Can you work these out from the model? Positions are in its coordinate system, mm. A direction names the side the tool comes from. Give positions to 0.01 mm unless a question says otherwise; leave off trailing zeros. Order: outer loops, then holes, each group sorted by start corner. A loop starts at its lowest first (then second) coordinate and runs counter-clockwise, first axis right, second up. Notation, with made-up numbers: (58.5, 44.25) - (84.5, 44.25) arc R12 ccw to (84.5, 62.25) - close; hole circle Ø4 at (-30, 40.5). An arc over 180 degrees is marked (long way). Answer as a JSON object with one key per item and string values.
```python
from build123d import *

# Parameters (mm, degrees)
SKETCH_1_R      = 45.75
SKETCH_1_R_2    = 1.5
EXTRUDE_1_DEPTH = 4


with BuildPart() as part:
    # 草图1 → 凸台-拉伸1 (new body)
    with BuildSketch(Plane(origin=(0, 0, 0), x_dir=(1, 0, 0), z_dir=(0, 1, 0))):
        with BuildLine():
            Line((-60, -10.5), (-60, 10.5))
            ThreePointArc((-60, 10.5), (-59.560660172, 11.560660172), (-58.5, 12))
            Line((-58.5, 12), (-54.863466897, 12))
            ThreePointArc((-54.863466897, 12), (-53.938159008, 12.31940468), (-53.406914679, 13.14159292))
            ThreePointArc((-53.406914679, 13.14159292), (0, 55), (53.406914679, 13.14159292))
            ThreePointArc((53.406914679, 13.14159292), (53.938159008, 12.31940468), (54.863466897, 12))
            Line((54.863466897, 12), (58.5, 12))
            ThreePointArc((58.5, 12), (59.560660172, 11.560660172), (60, 10.5))
            Line((60, 10.5), (60, -10.5))
            ThreePointArc((60, -10.5), (59.560660172, -11.560660172), (58.5, -12))
            Line((58.5, -12), (54.863466897, -12))
            ThreePointArc((54.863466897, -12), (53.938159008, -12.31940468), (53.406914679, -13.14159292))
            ThreePointArc((53.406914679, -13.14159292), (0, -55), (-53.406914679, -13.14159292))
            ThreePointArc((-53.406914679, -13.14159292), (-53.938159008, -12.31940468), (-54.863466897, -12))
            Line((-54.863466897, -12), (-58.5, -12))
            ThreePointArc((-58.5, -12), (-59.560660172, -11.560660172), (-60, -10.5))
        make_face()
        with Locations(Location((0, 0, 0), (0, 0, 270))):
            Circle(SKETCH_1_R, mode=Mode.SUBTRACT)
        with Locations(Location((0, 52.5, 0), (0, 0, 270))):
            Circle(SKETCH_1_R_2, mode=Mode.SUBTRACT)
        with Locations(Location((45.466333699, 26.25, 0), (0, 0, 270))):
            Circle(SKETCH_1_R_2, mode=Mode.SUBTRACT)
        with Locations(Location((45.466333699, -26.25, 0), (0, 0, 270))):
            Circle(SKETCH_1_R_2, mode=Mode.SUBTRACT)
        with Locations(Location((0, -52.5, 0), (0, 0, 270))):
            Circle(SKETCH_1_R_2, mode=Mode.SUBTRACT)
        with Locations(Location((-45.466333699, -26.25, 0), (0, 0, 270))):
            Circle(SKETCH_1_R_2, mode=Mode.SUBTRACT)
        with Locations(Location((-45.466333699, 26.25, 0), (0, 0, 270))):
            Circle(SKETCH_1_R_2, mode=Mode.SUBTRACT)
        with Locations(Location((-57.5, 9, 0), (0, 0, 270))):
            Circle(SKETCH_1_R_2, mode=Mode.SUBTRACT)
        with Locations(Location((57.5, 9, 0), (0, 0, 90))):
            Circle(SKETCH_1_R_2, mode=Mode.SUBTRACT)
        with Locations(Location((57.5, -9, 0), (0, 0, 270))):
            Circle(SKETCH_1_R_2, mode=Mode.SUBTRACT)
        with Locations(Location((-57.5, -9, 0), (0, 0, 90))):
            Circle(SKETCH_1_R_2, mode=Mode.SUBTRACT)
    extrude(amount=EXTRUDE_1_DEPTH)


solid = part.part
```
Q1. I need wall thicknesses on L1, parallel to X at y = 1.85, z = 0; L2, parallel to X at y = 2.9, z = 26.25; L3, parallel to X at y = 2.4, z = -27. Which ranges of each line are inside material? Lowest first, please.
Recorded:
{"L1": "x = -60 to -45.75, 45.75 to 60", "L2": "x = -48.33 to -46.97, -43.97 to -37.47, 37.47 to 43.97, 46.97 to 48.33", "L3": "x = -47.92 to -46.77, -44.17 to -36.93, 36.93 to 44.17, 46.77 to 47.92"}
Q2. If we section it at B-B, the plane z = 3: Please give me the cut outline in (x, y).
Recorded:
{"outline": "(-60, 0) - (-45.65, 0) - (-45.65, 4) - (-60, 4) - close; (45.65, 0) - (60, 0) - (60, 4) - (45.65, 4) - close"}
Q3. If we section it at C-C, the plane z = -9: Please give me the cut outline in (x, y).
Recorded:
{"outline": "(-60, 0) - (-59, 0) - (-59, 4) - (-60, 4) - close; (-56, 0) - (-44.86, 0) - (-44.86, 4) - (-56, 4) - close; (44.86, 0) - (56, 0) - (56, 4) - (44.86, 4) - close; (59, 0) - (60, 0) - (60, 4) - (59, 4) - close"}
Q4. If we section it at D-D, the plane y = 2.9: Count the separate pieces of the cut face and the enclosed holes in it, then the cut area to 3 significant figures.
Recorded:
{"separate pieces": "1", "enclosed holes": "11", "area": "3,120 mm^2"}
Q5. I'm going to push flat-ended pins straight in: pin 1 Ø1.8 at (x, y) = (56, 1.5) entering from -Z; pin 2 Ø1 at (x, y) = (-32, 2.5) entering from -Z; pin 3 Ø2 at (y, z) = (1.5, -15) entering from +X. Where does each tip first touch, or does it pass through?
Recorded:
{"pin 1": "stops at z = -12", "pin 2": "stops at z = -45.09", "pin 3": "stops at x = 53.19"}
Q6. Which directions (+Z, -Z, +X, -X, +Y, -Y) give clear straight access to the entire face, cutting with the end or side of a thin tool? Please do faces 4 (the face through (60, 2, 0)), 5 (the face through (-57, 2, 12)), 6 (the face through (-57, 2, -12)).
Recorded:
{"face 4": "+Z, -Z, +X, +Y, -Y", "face 5": "+Z, -X, +Y, -Y", "face 6": "-Z, -X, +Y, -Y"}
Q7. We'd pull the mould along Z, two halves only. Please class faces 1 (the face through (57, 2, 12)), 2 (the face through (23, 0, 40)), 3 (the face through (59, 2, 9)): released by +Z, released by -Z, zero draft, split by the parting line, or undercut.
Recorded:
{"face 1": "released by +Z", "face 2": "zero draft", "face 3": "undercut"}
Q8. If we section it at A-A, the plane x = 5: Please give me the cut outline in (y, z), then the cut area to 3 significant figures.
Recorded:
{"outline": "(0, -54.77) - (4, -54.77) - (4, -45.48) - (0, -45.48) - close; (0, 45.48) - (4, 45.48) - (4, 54.77) - (0, 54.77) - close", "area": "74.4 mm^2"}
